Part model, mm, in its own coordinate system. Face numbers are marked on the shaded views. A direction names the side the tool comes from. Coordinates: 2 decimals unless noted, no trailing zeros. Loops run counter-clockwise (first coordinate to the right, second up) from the corner with the lowest first, then second, coordinate; pieces in that order, holes last. Notation, with made-up numbers: M 38.5,11.25 L 63.5,11.25 A31 cw 63.5,48.25 Z; hole C 63.25,16 d7. An arc over 180 degrees is marked long. Use CSV: the item, a comma, the result in double quotes. Start each with the question number.
from build123d import *

# Parameters (mm, degrees)
F2_R      = 2
F3_DEPTH  = 10
F3_FACE_R = 2
F2_R_2    = 5
F2_R_3    = 4
F4_DEPTH  = 7.6
F5_DEPTH  = 25


with BuildPart() as f1:
    # F0 (on Right) → F1 (revolve)
    with BuildSketch(Plane.YZ):
        with BuildLine():
            Line((-2, 0), (0, 0))
            Line((0, 0), (0, 23))
            ThreePointArc((0, 23), (-0.8786796564, 25.1213203436), (-3, 26))
            Line((-3, 26), (-40, 26))
            Line((-40, 26), (-40, 24))
            Line((-40, 24), (-44.203865394, 24))
            ThreePointArc((-44.203865394, 24), (-44.9109721752, 23.7071067812), (-45.203865394, 23))
            Line((-45.203865394, 23), (-45.203865394, 22.5))
            Line((-45.203865394, 22.5), (-35.203865394, 22.5))
            Line((-35.203865394, 22.5), (-29.6515244991, 24))
            Line((-29.6515244991, 24), (-3, 24))
            ThreePointArc((-3, 24), (-2.2928932188, 23.7071067812), (-2, 23))
            Line((-2, 23), (-2, 0))
        make_face()
    revolve(axis=Axis((0, -18.7915153801, 0), (0, 1, 0)))

    # F2 (on face) → F3 (join)
    with BuildSketch(Plane(origin=(0, 0, 0), x_dir=(-1, 0, 0), z_dir=(0, 1, 0))):
        with BuildLine():
            ThreePointArc((22.6, -4.2708313008), (24.3588989435, -2.4494897428), (25, 0))
            ThreePointArc((25, 0), (24.3588989435, 2.4494897428), (22.6, 4.2708313008))
            ThreePointArc((22.6, 4.2708313008), (22.8997816583, 2.144761059), (23, 0))
            ThreePointArc((23, 0), (22.8997816583, -2.144761059), (22.6, -4.2708313008))
        make_face()
        with BuildLine():
            ThreePointArc((23, 0), (22.8997816583, 2.144761059), (22.6, 4.2708313008))
            ThreePointArc((22.6, 4.2708313008), (15, 0), (22.6, -4.2708313008))
            ThreePointArc((22.6, -4.2708313008), (22.8997816583, -2.144761059), (23, 0))
        make_face()
        with Locations((20, 0)):
            Circle(F2_R, mode=Mode.SUBTRACT)
        with BuildLine():
            ThreePointArc((-15, 0), (-17.5505102572, 4.3588989435), (-22.6, 4.2708313008))
            ThreePointArc((-22.6, 4.2708313008), (-23, 0), (-22.6, -4.2708313008))
            ThreePointArc((-22.6, -4.2708313008), (-17.5505102572, -4.3588989435), (-15, 0))
        make_face()
        with Locations((-20, 0)):
            Circle(F2_R, mode=Mode.SUBTRACT)
        with BuildLine():
            ThreePointArc((-22.6, -4.2708313008), (-23, 0), (-22.6, 4.2708313008))
            ThreePointArc((-22.6, 4.2708313008), (-25, 0), (-22.6, -4.2708313008))
        make_face()
    extrude(amount=-F3_DEPTH)

    # F3_face (on face) + F2 (on face) + F3_face1 (on face) → F4 (cut)
    with BuildSketch(Plane(origin=(-20, -2, 0), x_dir=(1, 0, 0), z_dir=(0, -1, 0))):
        Circle(F3_FACE_R)
        with Locations((40, 0)):
            Circle(F3_FACE_R)
    with BuildSketch(Plane(origin=(0, 0, 0), x_dir=(-1, 0, 0), z_dir=(0, 1, 0))):
        with Locations((20, 0)):
            Circle(F2_R_2)
        with Locations((20, 0)):
            Circle(F2_R, mode=Mode.SUBTRACT)
        with Locations((-20, 0)):
            Circle(F2_R_2)
        with Locations((-20, 0)):
            Circle(F2_R, mode=Mode.SUBTRACT)
        with Locations((0, 16.4260324091)):
            Circle(F2_R_3)
    with BuildSketch(Plane(origin=(0, 0, 0), x_dir=(-1, 0, 0), z_dir=(0, 1, 0))):
        with BuildLine():
            ThreePointArc((0, 23), (-14.6760158095, 17.7091659871), (-22.6, 4.2708313008))
            ThreePointArc((-22.6, 4.2708313008), (-25, 0), (-22.6, -4.2708313008))
            ThreePointArc((-22.6, -4.2708313008), (0, -23), (22.6, -4.2708313008))
            ThreePointArc((22.6, -4.2708313008), (25, 0), (22.6, 4.2708313008))
            ThreePointArc((22.6, 4.2708313008), (14.6760158095, 17.7091659871), (0, 23))
        make_face()
    extrude(amount=-F4_DEPTH, dir=(0, -1, 0), mode=Mode.SUBTRACT)

    # F2 (on face) → F5 (cut)
    with BuildSketch(Plane(origin=(0, 0, 0), x_dir=(-1, 0, 0), z_dir=(0, 1, 0))):
        with Locations((0, 16.4260324091)):
            Circle(F2_R_3)
    extrude(amount=-F5_DEPTH, mode=Mode.SUBTRACT)


solid = f1.part
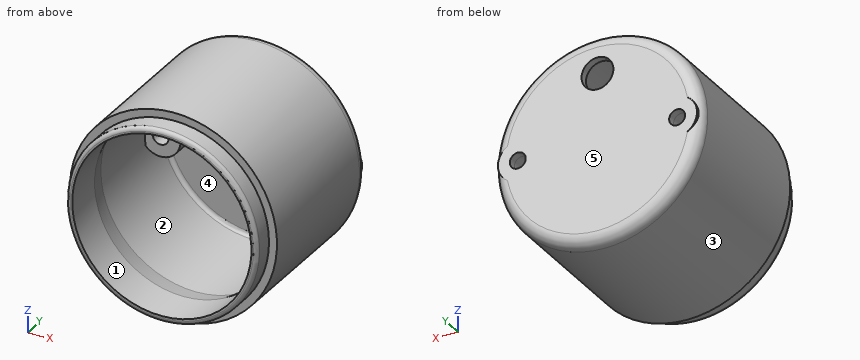
1. Slice it at B-B, the plane y = -39. List the corners of the cut face in (x, z).
2. Tool access for the marked faces 1 and 2: list every direction of +Z, -Z, +X, -X, +Y, -Y with a clear straight run to the whole face (end or side of a thin tool).
3. Pin check, flat tips, straight feed: pin 1 (4.5 mm diameter, centred on x = -20, z = 0, fed in from -Y); pin 2 (1.5 mm diameter, centred on x = -4.5, y = -18.5, fed in from +Z); pin 3 (10 mm diameter, centred on x = 9, z = -9, fed in from -Y); pin 4 (3.5 mm diameter, centred on x = 20, z = 0, fed in from -Y). Stop position of each tip, or through.
4. Two-plate mould, pull along Z, no slides. Class the marked faces 3, 4 and 5: pulls with the +Z half, pulls with the -Z half, needs draft (parallel to the pull), parting line crosses it, or undercut.
5. Slice it at D-D, the plane y = -20.5. List the corners of the cut face in (x, z).
6. Wall check: probe 1 along X at (y, z) = (-23.5, 0); probe 2 along Y at (x, z) = (12, -17); probe 3 along X at (y, z) = (-42, 0). Give the ranges that are in metal, low to high.
7. Slice it at C-C, the plane z = 1. State how many separate pieces and enclosed holes the cut face has, and give its area (3 significant figures).
8. Slice it at A-A, the plane x = 0. List the corners of the cut face in (y, z).
Found:
1,outline,"C 0,0 d52; hole C 0,0 d45"
2,face 1,"-Y"
2,face 2,"none"
3,pin 1,"y = -10"
3,pin 2,"z = 25.73"
3,pin 3,"y = -2"
3,pin 4,"through"
4,face 3,"parting line crosses it"
4,face 4,"undercut"
4,face 5,"needs draft"
5,outline,"C 0,0 d52; hole C 0,0 d48"
6,probe 1,"-26 to -24, 24 to 26"
6,probe 2,"-2 to 0"
6,probe 3,"-24 to -22.5, 22.5 to 24"
7,separate pieces,"3"
7,enclosed holes,"0"
7,area,"364 mm^2"
8,outline,"M -45.2,-23 A1 ccw -44.2,-24 L -40,-24 L -40,-26 L -3,-26 A3 ccw 0,-23 L 0,12.43 L -2,12.43 L -2,-23 A1 cw -3,-24 L -29.65,-24 L -35.2,-22.5 L -45.2,-22.5 Z; M -45.2,22.5 L -35.2,22.5 L -29.65,24 L -3,24 A1 cw -2,23 L -2,20.43 L 0,20.43 L 0,23 A3 ccw -3,26 L -40,26 L -40,24 L -44.2,24 A1 ccw -45.2,23 Z"
